Work out the finished part from the listing and answer in its coordinate system (mm). A direction names the side the tool comes from. Coordinates: 2 decimals unless noted, no trailing zeros. Order: outer loops, then holes, each group sorted by start corner. A loop starts at its lowest first (then second) coordinate and runs counter-clockwise, first axis right, second up. Notation, with made-up numbers: (81.5, -9.5) - (92.5, -9.5) arc R7 ccw to (92.5, 0.5) - close; hole circle Ø4 at (10, 83.25). An arc over 180 degrees is marked (long way). Answer as a JSON object with one key per item and string values. Group by question number.
1) Section B-B (y = 7.5) is taken. Give the vertices of the cut face in (x, z), plus the area to 3 significant figures.
2) Section C-C (x = -9) is taken. Give the vertices of the cut face in (y, z), plus the area to 3 significant figures.
3) Section D-D (y = -44.5) is taken. Give the vertices of the cut face in (x, z).
4) A tool of negligible diameter and unlimited length cuts with its end or side. For faces 1 (the face through (-377, -1, -125)), 2 (the face through (-450.858, 52.747, -98.823)), from which of +Z, -Z, +X, -X, +Y, -Y can it reach the whole face along a straight path? Write none if from no direction.
5) The mould has two halves that part along X. Classify faces 3 (the face through (-2, 61.912, 12)), 4 (the face through (5, -1, 0)), 5 (the face through (-450.38, -1.13, 73.86)): released by +X, released by -X, zero draft, split by the parting line, or undercut.
6) Find the intervals of material crossed by line 1 along X through (y, z) = (30, -14); line 2 along X through (y, z) = (44, -68.5); line 3 along Z through (x, y) = (-146.5, -16.5), in increasing order.
7) This flat-tipped pin is pushed along its axis until it touches: P1, Ø3, axis at x = 230, y = 21.5, coming from the -Z side. Where does it stop, or does it pass through?
8) Section A-A (z = -97.5) is taken. Give the vertices of the cut face in (x, y), plus the area to 3 significant figures.
from build123d import *

# Parameters (mm, degrees)
BOSS_EXTRUDE1_DEPTH      = 61.9125
BOSS_EXTRUDE1_DEPTH_BACK = 65.0875
FILLET1_R                = 30.48


with BuildPart() as part:
    # Sketch1 → Boss-Extrude1 (new body, two sides)
    with BuildSketch(Plane(origin=(0, 0, 0), x_dir=(1, 0, 0), z_dir=(0, 1, 0))) as boss_extrude1_sk:
        Polygon((376.9999953, 0), (-376.9999953, 0), (-376.9999953, 254), (-459.5499953, 254), (-459.5499953, -82.55), (459.5499953, -82.55), (459.5499953, 254), (376.9999953, 254), align=None)
    extrude(amount=BOSS_EXTRUDE1_DEPTH)
    extrude(boss_extrude1_sk.sketch, amount=-BOSS_EXTRUDE1_DEPTH_BACK)

    # Fillet1
    fillet1_edges = [part.edges().sort_by_distance(p)[0] for p in [
        (459.5499953, -1.5875, 82.55),
        (-459.5499953, -1.5875, 82.55),
        (-459.5499953, -65.0875, -85.725),
        (-459.5499953, 61.9125, -85.725),
        (0, -65.0875, 82.55),
        (0, 61.9125, 82.55),
        (459.5499953, 61.9125, -85.725),
        (459.5499953, -65.0875, -85.725),
    ]]
    fillet(fillet1_edges, radius=FILLET1_R)


solid = part.part
Report:
{
 "1": {"outline": "(-459.55, -254) - (-377, -254) - (-377, 0) - (377, 0) - (377, -254) - (459.55, -254) - (459.55, 52.07) arc R30.48 ccw to (429.07, 82.55) - (-429.07, 82.55) arc R30.48 ccw to (-459.55, 52.07) - close", "area": "117,000 mm²"},
 "2": {"outline": "(-65.09, 0) - (61.91, 0) - (61.91, 52.07) arc R30.48 ccw to (31.43, 82.55) - (-34.61, 82.55) arc R30.48 ccw to (-65.09, 52.07) - close", "area": "10,100 mm²"},
 "3": {"outline": "(-457.9, -254) - (-377, -254) - (-377, 0) - (377, 0) - (377, -254) - (457.9, -254) - (457.9, 52.07) arc R28.83 ccw to (429.07, 80.9) - (-429.07, 80.9) arc R28.83 ccw to (-457.9, 52.07) - close"},
 "4": {"face 1": "-Z, +Y, -Y", "face 2": "+Z, -Z, -X, +Y"},
 "5": {"face 3": "zero draft", "face 4": "undercut", "face 5": "released by -X"},
 "6": {"line 1": "x = -459.55 to -377, 377 to 459.55", "line 2": "x = -456.84 to -377, 377 to 456.84", "line 3": "z = 0 to 82.55"},
 "7": {"P1": "stops at z = 0"},
 "8": {"outline": "(-459.55, -34.61) arc R30.48 ccw to (-429.07, -65.09) - (-377, -65.09) - (-377, 61.91) - (-429.07, 61.91) arc R30.48 ccw to (-459.55, 31.43) - close; (377, -65.09) - (429.07, -65.09) arc R30.48 ccw to (459.55, -34.61) - (459.55, 31.43) arc R30.48 ccw to (429.07, 61.91) - (377, 61.91) - close", "area": "20,200 mm²"}
}
